from build123d import *

# Parameters (mm, degrees)
F11_DEPTH = 5.59188
F4_R      = 1.3
F5_R      = 1.3
F9_R      = 1.3
F6_R      = 1.3
F10_R     = 1.3
F12_DEPTH = 12.5
F13_R     = 5
F14_R     = 7


with BuildPart() as f11:
    # F0 (on Front) → F11 (new body)
    with BuildSketch(Plane.XZ):
        with BuildLine():
            Line((5.074043, 125.446646), (-18.925957, 125.446646))
            Line((-18.925957, 125.446646), (-18.925957, -30.753354))
            Line((-18.925957, -30.753354), (13.074043, -30.753354))
            Line((13.074043, -30.753354), (13.074043, -32.253354))
            Line((13.074043, -32.253354), (10.574043, -32.253354))
            Line((10.574043, -32.253354), (10.574043, -38.253354))
            Line((10.574043, -38.253354), (17.939503, -32.253354))
            Line((17.939503, -32.253354), (17.939503, -21.653354))
            Line((17.939503, -21.653354), (0, -21.653354))
            ThreePointArc((0, -21.653354), (-5.66883, -17.703115), (-3.925964, -11.017126))
            ThreePointArc((-3.925964, -11.017126), (0.25929, -3.046463), (-3.820934, 4.978473))
            ThreePointArc((-3.820934, 4.978473), (-6.236981, 13.558536), (-2.382879, 21.59599))
            ThreePointArc((-2.382879, 21.59599), (-0.24316, 30.291685), (-3.820934, 38.501012))
            ThreePointArc((-3.820934, 38.501012), (-8.035456, 46.644288), (-3.820934, 54.787565))
            ThreePointArc((-3.820934, 54.787565), (0.543337, 62.931922), (-4.625957, 70.590631))
            ThreePointArc((-4.625957, 70.590631), (-7.774459, 76.938306), (-4.625957, 83.285981))
            ThreePointArc((-4.625957, 83.285981), (1.031725, 93.12844), (-4.625957, 102.970899))
            ThreePointArc((-4.625957, 102.970899), (-7.063194, 107.892131), (-4.625957, 112.813362))
            ThreePointArc((-4.625957, 112.813362), (2.40535, 117.455168), (5.074043, 125.446646))
        make_face()
    extrude(amount=F11_DEPTH)

    # F4 (on face) + F5 (on face) + F9 (on face) + F6 (on face) + F10 (on face) → F12 (cut, symmetric)
    with BuildSketch(Plane(origin=(0, -0.41406, -0.097651), x_dir=(-1, 0, 0), z_dir=(0, 0.973299, 0.22954))):
        with Locations((4.625957, -1.803868)):
            Circle(F4_R)
    with BuildSketch(Plane(origin=(0, 6.556371, 1.546236), x_dir=(-1, 0, 0), z_dir=(0, 0.973299, 0.22954))):
        with Locations((4.625957, 28.563067)):
            Circle(F5_R)
    with BuildSketch(Plane(origin=(0, 20.497232, 4.83401), x_dir=(-1, 0, 0), z_dir=(0, 0.973299, 0.22954))):
        with Locations((4.625957, 89.296936)):
            Circle(F9_R)
    with BuildSketch(Plane(origin=(0, 13.526801, 3.190123), x_dir=(-1, 0, 0), z_dir=(0, 0.973299, 0.22954))):
        with Locations((4.625957, 58.930002)):
            Circle(F6_R)
    with BuildSketch(Plane(origin=(0, 27.467663, 6.477897), x_dir=(-1, 0, 0), z_dir=(0, 0.973299, 0.22954))):
        with Locations((4.625957, 119.663871)):
            Circle(F10_R)
    extrude(amount=F12_DEPTH, both=True, mode=Mode.SUBTRACT)

    # F13
    f13_edges = [f11.edges().sort_by_distance(p)[0] for p in [
        (17.939503, -2.79594, -21.653354),
    ]]
    fillet(f13_edges, radius=F13_R)

    # F14
    f14_edges = [f11.edges().sort_by_distance(p)[0] for p in [
        (17.939503, -2.79594, -32.253354),
    ]]
    fillet(f14_edges, radius=F14_R)


solid = f11.part
The model under review builds one solid part; all positions refer to its coordinate system, in mm. A direction names the side the tool comes from. Coordinates: 2 decimals unless noted, no trailing zeros. Loops run counter-clockwise (first coordinate to the right, second up) from the corner with the lowest first, then second, coordinate; pieces in that order, holes last. Notation, with made-up numbers: M 6.25,47.25 L 41.25,47.25 A28 ccw 41.25,82.25 Z; hole C 68.25,-9.5 d5. An arc over 180 degrees is marked long. Put each result on its own line as item: value. Start each with the question number.
Q1. Add section B-B (z = 13). Write out the cut boundary in (x, y), and give its area (3 significant figures).
Q2. Clearance check with flat-ended pins moving along their axes: pin 1 (3 mm diameter, centred on x = 5, y = -5, fed in from -Z); pin 2 (2 mm diameter, centred on x = 11.5, y = -3, fed in from +Z); pin 3 (1.7 mm diameter, centred on y = -2.5, z = -36, fed in from -X). State where each tip first meets the part, or that it passes through.
Q3. For faces 4 (the cylindrical face through (2.33, -2.76, 117.36)), 5 (the cylindrical face through (16.514, -2.835, -23.157)), 6 (the flat face through (10.574, -3, -35)), list the 3-axis set-ups (+Z, -Z, +X, -X, +Y, -Y) from which the entire face can be reached by the end or side of a thin tool; tool diameter is ignored.
Q4. Add section C-C (x = -13). Write out the cut boundary in (y, z).
Q5. Wall thickness on line 1 (X direction, y = -0.55, z = 29); line 2 (Z direction, x = -10.5, y = -2.1); line 3 (Z direction, x = -1.5, y = -4.35): over which ranges is each line inside the solid? List them lowest first.
Q6. The part is to be moulded in two halves that separate along Z. For faces 1 (the flat face through (-7, -3, 125.447)), 2 (the flat face through (7, -3, -21.653)), 3 (the cylindrical face through (17.28, -2.84, -31.89)), say which applies: +Z half, -Z half, draft (parallel to the pull), parting line (faces both ways), or undercut.
Q7. Add section D-D (y = -2.5). Count the separate pieces of the cut face and the enclosed holes in it, and give its area (3 significant figures).
Q8. Add section A-A (x = 2.5). Write out the cut boundary in (y, z), and give its area (3 significant figures).
Answers:
1. outline: M -18.93,-5.59 L -6.27,-5.59 L -6.27,0 L -18.93,0 Z
1. area: 70.8 mm^2
2. pin 1: stops at z = -30.75
2. pin 2: stops at z = -21.65
2. pin 3: stops at x = 10.57
3. face 4: +X, +Y, -Y
3. face 5: +Z, +X, +Y, -Y
3. face 6: -Z, -X, +Y, -Y
4. outline: M -5.59,-30.75 L 0,-30.75 L 0,125.45 L -5.59,125.45 Z
5. line 1: x = -18.93 to -5.91, -3.34 to -0.19
5. line 2: z = -30.75 to 125.45
5. line 3: z = -30.75 to -21.46, -8.59 to 2.62, 23.21 to 35.01, 56.77 to 68.18, 85.97 to 100.29, 114.07 to 125.45
6. face 1: +Z half
6. face 2: undercut
6. face 3: -Z half
7. separate pieces: 1
7. enclosed holes: 5
7. area: 2,690 mm^2
8. outline: M -5.59,-30.75 L 0,-30.75 L 0,-21.65 L -5.59,-21.65 Z; M -5.59,117.58 L 0,117.58 L 0,125.45 L -5.59,125.45 Z
8. area: 94.9 mm^2
